from build123d import *

# Parameters (mm, degrees)
F3_R     = 2.8871491502
F4_DEPTH = 25


with BuildPart() as f2:
    # F2: sweep along a path in F1
    with BuildLine(Plane.XY) as f2_path:
        Line((10.6192948297, 0), (10.6192948297, 14.1305187717))
        Line((10.6192948297, 14.1305187717), (0, 14.1305187717))
    # F0 (on Front) → F2 (sweep)
    with BuildSketch(Plane.XZ):
        Polygon((10.6192948297, 10.8289821073), (10.6192948297, 0), (14.9371791631, 0), (14.9371791631, 13.4334210306), (8.6316959932, 13.4334210306), (8.6316959932, 12.2682768852), align=None)
    sweep(path=f2_path.line, transition=Transition.RIGHT)

    # F3 (on face) → F4 (cut)
    with BuildSketch(Plane.XY.offset(13.4334210306)):
        with Locations((8.6316959932, 12.1429199353)):
            Circle(F3_R)
    extrude(amount=-F4_DEPTH, mode=Mode.SUBTRACT)


solid = f2.part
Here's how the part is built. I have some questions about the finished solid (model axes, mm). A direction names the side the tool comes from. Round coordinates to 2 decimals unless told otherwise and drop trailing zeros. Loops run counter-clockwise (first coordinate to the right, second up) from the corner with the lowest first, then second, coordinate; pieces in that order, holes last. Notation, with made-up numbers: M -21,-21.5 L -5,-21.5 A33 ccw -5,8.5 Z; hole C 64.25,18.25 d3. An arc over 180 degrees is marked long. Write each question's results on one line, items separated by ' | '. Start each with the question number.
(1) Thinking about a two-plate mould opening in X: for faces 1 (the flat face through (9.61, 5.09, 11.56)), 2 (the cylindrical face through (10.739, 14.116, 6.811)), 3 (the flat face through (3, 12.143, 13)), which applies, pulls with the +X half, pulls with the -X half, needs draft (parallel to the pull), parting line crosses it, or undercut?
(2) I want a section at D-D (x = 1.5). Please give me the cut outline in (y, z).
(3) I want a section at C-C (y = 12.5). Please give me the cut outline in (x, z).
(4) I want a section at A-A (z = 5.5). Please give me the cut outline in (x, y).
(5) If I drill on probe 1 along X at (y, z) = (9, 8.75); probe 2 along X at (y, z) = (14.5, 3); probe 3 along X at (y, z) = (14.25, 6), over which ranges is the centre line in solid material (lowest first)? Write a range as from..to.
(6) Will these pins go through, and if not, where does the flat tip stop? P1, Ø6, axis at y = 4.5, z = 5.5, coming from the -X side; P2, Ø0.6, axis at y = 4, z = 13, coming from the -X side; P3, Ø5, axis at x = 2.5, z = 8, coming from the -Y side.
(7) I want a section at B-B (x = 9.75). Please give me the cut outline in (y, z).
(8) On a 3-axis mill with a long thin cutter (end or side, diameter ignored), from which of +Z, -Z, +X, -X, +Y, -Y can I reach the whole of each face in a straight line? I mean faces 4 (the flat face through (7, 18.448, 7)), 5 (the flat face through (8.632, 5, 13)), 6 (the flat face through (3, 14.131, 5)). Say none if no direction works.
Solved:
1) face 1: pulls with the -X half | face 2: undercut | face 3: needs draft
2) outline: M 12.14,12.27 L 14.13,10.83 L 14.13,0 L 18.45,0 L 18.45,13.43 L 12.14,13.43 Z
3) outline: M 0,12.01 L 5.77,12.01 L 5.77,13.43 L 0,13.43 Z; M 11.5,0 L 14.94,0 L 14.94,13.43 L 11.5,13.43 Z
4) outline: M 0,14.13 L 6.54,14.13 A2.89 cw long 10.62,10.05 L 10.62,0 L 14.94,0 L 14.94,18.45 L 0,18.45 Z
5) probe 1: x = 10.62..14.94 | probe 2: x = 0..6.96, 10.3..14.94 | probe 3: x = 0..6.66, 10.61..14.94
6) P1: stops at x = 10.62 | P2: stops at x = 8.63 | P3: stops at y = 14.13
7) outline: M 0,11.46 L 9.48,11.46 L 9.48,13.43 L 0,13.43 Z; M 14.8,0 L 18.45,0 L 18.45,13.43 L 14.8,13.43 Z
8) face 4: +Z, -Z, +X, -X, +Y | face 5: +Z, -Z, -X, -Y | face 6: -Z, -X, -Y
